from build123d import *

# Parameters (mm, degrees)
SKETCH1_W           = 130
SKETCH1_H           = 104.86
BOSS_EXTRUDE1_DEPTH = 39.84
SKETCH2_W           = 130
SKETCH2_H           = 94.86
CUT_EXTRUDE1_DEPTH  = 6.6
SKETCH3_W           = 18.25
SKETCH3_H           = 89.15
CUT_EXTRUDE2_DEPTH  = 6.98
SKETCH5_W           = 50.415
SKETCH5_H           = 94.86
CUT_EXTRUDE3_DEPTH  = 20.6
SKETCH6_R           = 1.5
CUT_EXTRUDE4_DEPTH  = 12.4
SKETCH7_W           = 50.415
SKETCH7_H           = 20.5
CUT_EXTRUDE5_DEPTH  = 12.4
SKETCH9_W           = 23
SKETCH9_H           = 15
CUT_EXTRUDE7_DEPTH  = 12.4
CUT_EXTRUDE8_DEPTH  = 5
SKETCH11_R          = 1.5
CUT_EXTRUDE9_DEPTH  = 15
FILLET2_R           = 3.175
FILLET3_R           = 3.175
FILLET4_R           = 3.175
FILLET5_R           = 1.5875
FILLET6_R           = 3.175


with BuildPart() as part:
    # Sketch1 → Boss-Extrude1 (new body)
    with BuildSketch(Plane.XY):
        with Locations((65, -52.43)):
            Rectangle(SKETCH1_W, SKETCH1_H)
    extrude(amount=BOSS_EXTRUDE1_DEPTH)

    # Sketch2 → Cut-Extrude1 (cut)
    with BuildSketch(Plane.XY.offset(39.84)):
        with Locations((65, -47.43)):
            Rectangle(SKETCH2_W, SKETCH2_H)
    extrude(amount=-CUT_EXTRUDE1_DEPTH, mode=Mode.SUBTRACT)

    # Sketch3 → Cut-Extrude2 (cut)
    with BuildSketch(Plane.XY.offset(33.24)):
        with Locations((65, -44.575)):
            Rectangle(SKETCH3_W, SKETCH3_H)
    extrude(amount=-CUT_EXTRUDE2_DEPTH, mode=Mode.SUBTRACT)

    # Sketch5 → Cut-Extrude3 (cut)
    with BuildSketch(Plane.XY.offset(33.24)):
        with Locations((104.7925, -47.43)):
            Rectangle(SKETCH5_W, SKETCH5_H)
        with Locations((25.2075, -47.43)):
            Rectangle(SKETCH5_W, SKETCH5_H)
    extrude(amount=-CUT_EXTRUDE3_DEPTH, mode=Mode.SUBTRACT)

    # Sketch6 → Cut-Extrude4 (cut)
    with BuildSketch(Plane.XY.offset(12.64)):
        with Locations((35.925, -25.6)):
            Circle(SKETCH6_R)
        with Locations((6.925, -25.6)):
            Circle(SKETCH6_R)
        with Locations((35.925, -54.6)):
            Circle(SKETCH6_R)
        with Locations((6.925, -54.6)):
            Circle(SKETCH6_R)
        with Locations((94.075, -25.6)):
            Circle(SKETCH6_R)
        with Locations((123.075, -25.6)):
            Circle(SKETCH6_R)
        with Locations((94.075, -54.6)):
            Circle(SKETCH6_R)
        with Locations((123.075, -54.6)):
            Circle(SKETCH6_R)
    extrude(amount=-CUT_EXTRUDE4_DEPTH, mode=Mode.SUBTRACT)

    # Sketch7 → Cut-Extrude5 (cut)
    with BuildSketch(Plane.XY.offset(12.64)):
        with Locations((25.2075, -10.25)):
            Rectangle(SKETCH7_W, SKETCH7_H)
        with Locations((104.7925, -10.25)):
            Rectangle(SKETCH7_W, SKETCH7_H)
    extrude(amount=-CUT_EXTRUDE5_DEPTH, mode=Mode.SUBTRACT)

    # Sketch9 → Cut-Extrude7 (cut)
    with BuildSketch(Plane.XY.offset(12.64)):
        with Locations((108.575, -28)):
            Rectangle(SKETCH9_W, SKETCH9_H)
        with Locations((21.425, -28)):
            Rectangle(SKETCH9_W, SKETCH9_H)
    extrude(amount=-CUT_EXTRUDE7_DEPTH, mode=Mode.SUBTRACT)

    # Sketch10 → Cut-Extrude8 (cut)
    with BuildSketch(Plane.XY.offset(12.64)):
        Polygon((9.925, -28.6), (3, -28.6), (3, -51.6), (9.925, -51.6), (9.925, -61.6), (32.925, -61.6), (32.925, -51.6), (42.925, -51.6), (42.925, -28.6), (32.925, -28.6), (32.925, -35.5), (9.925, -35.5), align=None)
        Polygon((97.075, -28.6), (87.075, -28.6), (87.075, -51.6), (97.075, -51.6), (97.075, -61.6), (120.075, -61.6), (120.075, -51.6), (127, -51.6), (127, -28.6), (120.075, -28.6), (120.075, -35.5), (97.075, -35.5), align=None)
    extrude(amount=-CUT_EXTRUDE8_DEPTH, mode=Mode.SUBTRACT)

    # Sketch11 → Cut-Extrude9 (cut)
    with BuildSketch(Plane.XY.offset(33.24)):
        with Locations((53.145, -20)):
            Circle(SKETCH11_R)
        with Locations((76.855, -20)):
            Circle(SKETCH11_R)
        with Locations((53.145, -91)):
            Circle(SKETCH11_R)
        with Locations((76.855, -91)):
            Circle(SKETCH11_R)
    extrude(amount=-CUT_EXTRUDE9_DEPTH, mode=Mode.SUBTRACT)

    # Fillet2
    fillet2_edges = [part.edges().sort_by_distance(p)[0] for p in [
        (3, -51.6, 10.14),
    ]]
    fillet(fillet2_edges, radius=FILLET2_R)

    # Fillet3
    fillet3_edges = [part.edges().sort_by_distance(p)[0] for p in [
        (50.415, -20.5, 6.44),
        (79.585, -20.5, 6.44),
        (32.925, -35.5, 3.94),
        (9.925, -35.5, 3.94),
        (42.925, -28.6, 10.14),
        (42.925, -51.6, 10.14),
        (32.925, -61.6, 10.14),
        (9.925, -61.6, 10.14),
        (3, -28.6, 10.14),
        (127, -28.6, 10.14),
        (127, -51.6, 10.14),
        (120.075, -61.6, 10.14),
        (97.075, -61.6, 10.14),
        (87.075, -51.6, 10.14),
        (87.075, -28.6, 10.14),
    ]]
    fillet(fillet3_edges, radius=FILLET3_R)

    # Fillet4
    fillet4_edges = [part.edges().sort_by_distance(p)[0] for p in [
        (120.075, -35.5, 3.94),
        (97.075, -35.5, 3.94),
    ]]
    fillet(fillet4_edges, radius=FILLET4_R)

    # Fillet5
    fillet5_edges = [part.edges().sort_by_distance(p)[0] for p in [
        (74.125, -89.15, 29.75),
        (55.875, -89.15, 29.75),
    ]]
    fillet(fillet5_edges, radius=FILLET5_R)

    # Fillet6
    fillet6_edges = [part.edges().sort_by_distance(p)[0] for p in [
        (79.585, -94.86, 22.94),
        (50.415, -94.86, 22.94),
    ]]
    fillet(fillet6_edges, radius=FILLET6_R)


solid = part.part
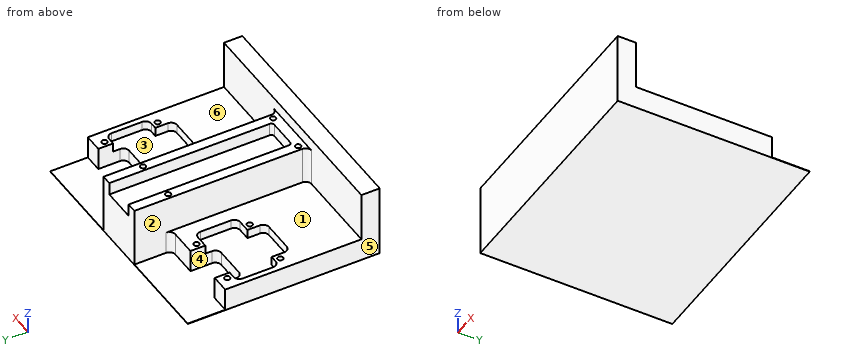
Input: part model. Units: mm. Frame: model coordinates. Face numbers are marked on the shaded views. A direction names the side the tool comes from. Coordinates: 2 decimals unless noted, no trailing zeros. Order: outer loops, then holes, each group sorted by start corner. A loop starts at its lowest first (then second) coordinate and runs counter-clockwise, first axis right, second up. Notation, with made-up numbers: M 83,-15.75 L 90,-15.75 A23 cw 90,12.25 Z; hole C 12.5,7 d4. An arc over 180 degrees is marked long. Answer in a Markdown table with one row per item.
(1) Draft query along X for the marked faces 1, 2 and 3. Return one class per face: pulls with the +X half, pulls with the -X half, needs draft (parallel to the pull), parting line crosses it, or undercut.
Numbers:
| item | result |
|---|---|
| face 1 | needs draft |
| face 2 | pulls with the -X half |
| face 3 | undercut |
(2) Section query A-A, the plane z = 30.5. Give the number of separate pieces and of enclosed holes in the cut face, plus the area to 3 significant figures.
Numbers:
| item | result |
|---|---|
| separate pieces | 1 |
| enclosed holes | 4 |
| area | 2,420 mm^2 |
(3) Material intervals for line 1 (Z direction, x = 76, y = -88); line 2 (Y direction, x = 108, z = 22); line 3 (Z direction, x = 98.5, y = -28), sorted ascending. Write a range as [from, to].
Numbers:
| item | result |
|---|---|
| line 1 | z = [0, 33.24] |
| line 2 | y = [-104.86, -94.86] |
| line 3 | z = [0, 0.24] |
(4) Contact query for flat-ended pins moving along their axis: pin 1 Ø5.5 at (x, z) = (24, 10) entering from +Y; pin 2 Ø12 at (x, y) = (67.5, -40.5) entering from +Z; pin 3 Ø4 at (x, z) = (36, 9.5) entering from +Y. Output: stop coordinate, or through.
Numbers:
| item | result |
|---|---|
| pin 1 | stops at y = -35.5 |
| pin 2 | stops at z = 26.26 |
| pin 3 | stops at y = -20.5 |
(5) Access query for the marked faces 4, 5 and 6. Directions: +Z, -Z, +X, -X, +Y, -Y. A direction counts if a zero-diameter tool reaches every point of the face in a straight line with its end or side. Return the directions, or none.
Numbers:
| item | result |
|---|---|
| face 4 | +Z, +Y |
| face 5 | +Z, -Z, -X, +Y, -Y |
| face 6 | +Z, +X, +Y |
(6) Section query B-B, the plane y = -85. Output: boundary loops of the cut face in (x, z) (3 decimals), plus the area to 3 significant figures.
Numbers:
| item | result |
|---|---|
| outline | M 0,0 L 130,0 L 130,12.64 L 79.585,12.64 L 79.585,33.24 L 74.125,33.24 L 74.125,26.26 L 55.875,26.26 L 55.875,33.24 L 50.415,33.24 L 50.415,12.64 L 0,12.64 Z |
| area | 2,120 mm^2 |
(7) Section query D-D, the plane z = 15. Output: boundary loops of the cut face in (x, y) (3 decimals), plus the area to 3 significant figures.
Numbers:
| item | result |
|---|---|
| outline | M 0,-104.86 L 130,-104.86 L 130,-94.86 L 82.76,-94.86 A3.175 cw 79.585,-91.685 L 79.585,0 L 50.415,0 L 50.415,-91.685 A3.175 cw 47.24,-94.86 L 0,-94.86 Z |
| area | 4,070 mm^2 |
